Input: part model. Units: mm. Frame: model coordinates. A direction names the side the tool comes from. Coordinates: 2 decimals unless noted, no trailing zeros. Loops run counter-clockwise (first coordinate to the right, second up) from the corner with the lowest first, then second, coordinate; pieces in that order, holes last. Notation, with made-up numbers: (72, 5.5) -> (112, 5.5) arc R5 cw to (112, 9.5) -> close; hole circle Ø9 at (-14, -29). An arc over 180 degrees is marked (long way). Answer as a JSON object with one key per item and string values.
from build123d import *

# Parameters (mm, degrees)
SKETCH1_W           = 25.4
SKETCH1_H           = 25.4
BOSS_EXTRUDE1_DEPTH = 1.6
SKETCH2_R           = 4.45
CUT_EXTRUDE1_DEPTH  = 19.031638861
CUT_EXTRUDE2_DEPTH  = 19.031638861
SKETCH4_W           = 25.4
SKETCH4_H           = 25.4
SKETCH4_R           = 1.0922
SKETCH4_R_2         = 4.45
BOSS_EXTRUDE2_DEPTH = 5.35


with BuildPart() as part:
    # Sketch1 → Boss-Extrude1 (new body)
    with BuildSketch(Plane.XY):
        Rectangle(SKETCH1_W, SKETCH1_H)
    extrude(amount=BOSS_EXTRUDE1_DEPTH)

    # Sketch2 → Cut-Extrude1 (cut, through all)
    with BuildSketch(Plane.XY.offset(1.6)):
        Circle(SKETCH2_R)
    extrude(amount=-CUT_EXTRUDE1_DEPTH, mode=Mode.SUBTRACT)

    # Sketch3 → Cut-Extrude2 (cut, through all)
    with BuildSketch(Plane.XY.offset(1.6)):
        Polygon((9.113937588, 5.861089595), (6.732687588, 5.861089595), (5.542062588, 7.923312588), (6.732687588, 9.985535581), (9.113937588, 9.985535581), (10.304562588, 7.923312588), align=None)
        Polygon((-6.732687588, 5.861089595), (-5.542062588, 7.923312588), (-6.732687588, 9.985535581), (-9.113937588, 9.985535581), (-10.304562588, 7.923312588), (-9.113937588, 5.861089595), align=None)
        Polygon((6.732687588, -5.861089595), (5.542062588, -7.923312588), (6.732687588, -9.985535581), (9.113937588, -9.985535581), (10.304562588, -7.923312588), (9.113937588, -5.861089595), align=None)
        Polygon((-9.113937588, -5.861089595), (-6.732687588, -5.861089595), (-5.542062588, -7.923312588), (-6.732687588, -9.985535581), (-9.113937588, -9.985535581), (-10.304562588, -7.923312588), align=None)
    extrude(amount=-CUT_EXTRUDE2_DEPTH, mode=Mode.SUBTRACT)

    # Sketch4 → Boss-Extrude2 (add)
    with BuildSketch(Plane(origin=(0, 0, 0), x_dir=(-1, 0, 0), z_dir=(0, 0, -1))):
        Rectangle(SKETCH4_W, SKETCH4_H)
        with Locations((7.923312588, -7.923312588)):
            Circle(SKETCH4_R, mode=Mode.SUBTRACT)
        with Locations((-7.923312588, -7.923312588)):
            Circle(SKETCH4_R, mode=Mode.SUBTRACT)
        with Locations((7.923312588, 7.923312588)):
            Circle(SKETCH4_R, mode=Mode.SUBTRACT)
        with Locations((-7.923312588, 7.923312588)):
            Circle(SKETCH4_R, mode=Mode.SUBTRACT)
        with Locations(Location((0, 0, 0), (0, 0, 180))):
            Circle(SKETCH4_R_2, mode=Mode.SUBTRACT)
    extrude(amount=BOSS_EXTRUDE2_DEPTH)


solid = part.part
1. Line query: line 1 along Y through (x, z) = (7.25, 0.75); line 2 along Y through (x, z) = (7.75, -1.25); line 3 along X through (y, z) = (0.25, 0.75). Output: solid intervals per line, ascending.
Reply:
{"line 1": "y = -12.7 to -9.99, -5.86 to 5.86, 9.99 to 12.7", "line 2": "y = -12.7 to -9, -6.84 to 6.84, 9 to 12.7", "line 3": "x = -12.7 to -4.44, 4.44 to 12.7"}
2. Section query B-B (x = 4). Return loops of the section in (y, z).
Reply:
{"outline": "(-12.7, -5.35) -> (-1.95, -5.35) -> (-1.95, 1.6) -> (-12.7, 1.6) -> close; (1.95, -5.35) -> (12.7, -5.35) -> (12.7, 1.6) -> (1.95, 1.6) -> close"}
3. Pin query (flat end, axial travel): P1, Ø7, axis at x = 0, y = 0, coming from the +Z side; P2, Ø1.2, axis at x = 7.5, y = -8.5, coming from the +Z side. Return the tip coordinate at first contact, or that it passes through.
Reply:
{"P1": "passes through", "P2": "stops at z = 0"}
4. Section query A-A (y = 0). Return loops of the section in (x, z).
Reply:
{"outline": "(-12.7, -5.35) -> (-4.45, -5.35) -> (-4.45, 1.6) -> (-12.7, 1.6) -> close; (4.45, -5.35) -> (12.7, -5.35) -> (12.7, 1.6) -> (4.45, 1.6) -> close"}
5. Mould query, pull axis Y, two halves, no side actions, for faces 3 (the face through (0, -12.7, -2)), 4 (the face through (0, 6, 1.6)), 5 (the face through (-9.72, -6.91, 0.81)). Classes: pulls with the +Y half, pulls with the -Y half, needs draft (parallel to the pull), parting line crosses it, or undercut.
Reply:
{"face 3": "pulls with the -Y half", "face 4": "needs draft", "face 5": "undercut"}
6. Section query D-D (z = 0.5). Count the separate pieces of the cut face and the enclosed holes in it, plus the area to 3 significant figures.
Reply:
{"separate pieces": "1", "enclosed holes": "5", "area": "524 mm2"}
7. Access query for faces 1 (the face through (7, 7, 0)), 2 (the face through (-5, 0, -5.35)). Directions: +Z, -Z, +X, -X, +Y, -Y. A direction counts if a zero-diameter tool reaches every point of the face in a straight line with its end or side. Return the directions, or none.
Reply:
{"face 1": "+Z", "face 2": "-Z, +X, -X, +Y, -Y"}
8. Section query C-C (z = -4.5). Return loops of the section in (x, y).
Reply:
{"outline": "(-12.7, -12.7) -> (12.7, -12.7) -> (12.7, 12.7) -> (-12.7, 12.7) -> close; hole circle Ø2.18 at (-7.92, -7.92); hole circle Ø2.18 at (-7.92, 7.92); hole circle Ø8.9 at (0, 0); hole circle Ø2.18 at (7.92, -7.92); hole circle Ø2.18 at (7.92, 7.92)"}
